Drawing for the job (mm, zero at the part's lowest x, y, z). A direction names the side the tool comes from. Round coordinates to 2 decimals unless told otherwise and drop trailing zeros. Write each loop counter-clockwise with the first axis right and the second up, starting at its lowest first coordinate (ties: lowest second). Pieces come first, ordered by that corner, then holes.
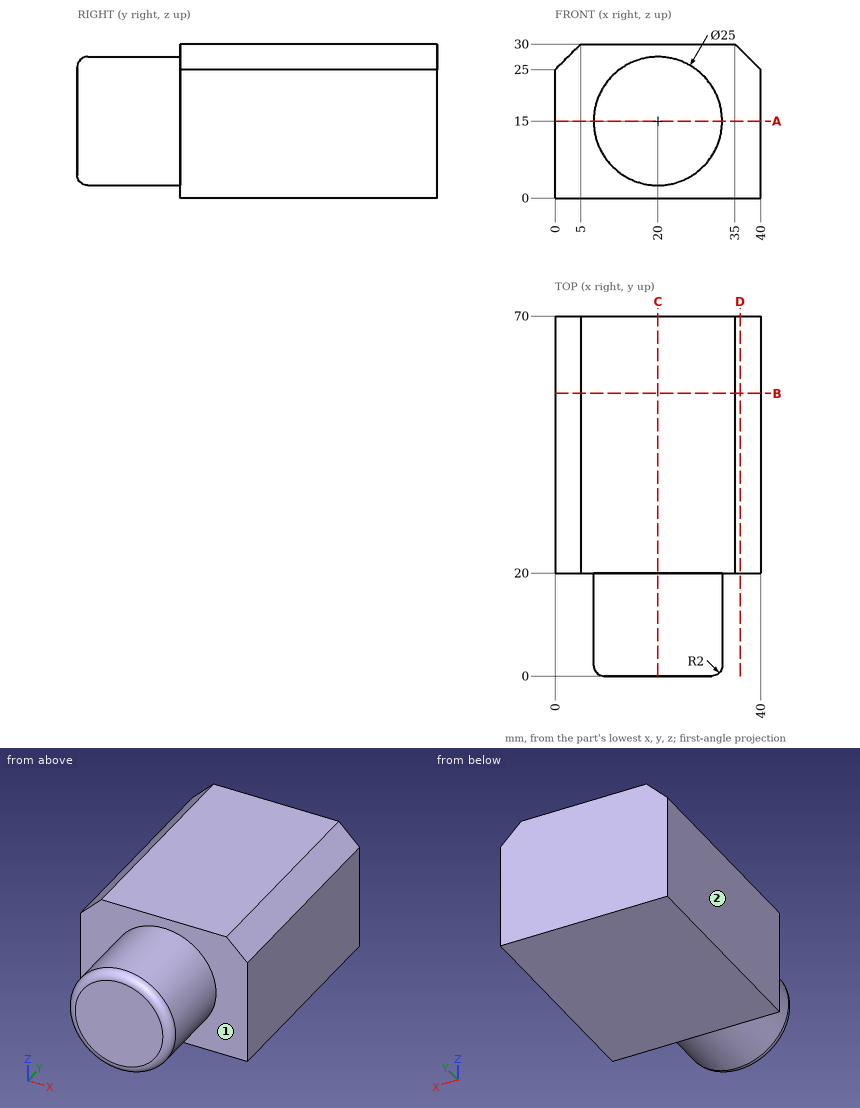
Q1. Tool access for the marked faces 1 and 2: list every direction of +Z, -Z, +X, -X, +Y, -Y with a clear straight run to the whole face (end or side of a thin tool).
Q2. Drop a flat-ended pin along its axis: P1, Ø1, axis at y = 7.5, z = 11.5, coming from the -X side. Give the stop position or say it passes through.
Q3. Saw through at D-D, the plane x = 36. Write the cut outline in (y, z), and give its area (3 significant figures).
Q4. Saw through at B-B, the plane y = 55. Write the cut outline in (x, z), and give its area (4 significant figures).
Q5. Saw through at A-A, the plane z = 15. Write the cut outline in (x, y), and give its area (3 significant figures).
Q6. Saw through at C-C, the plane x = 20. Write the cut outline in (y, z), and give its area (3 significant figures).
Q7. Wall check: line 1 (Y direction, x = 5, z = 7.75); line 2 (Y direction, x = 20.5, z = 26.5); line 3 (Z direction, x = 11.5, y = 10). Give the ranges that are in metal, low to high.
Computed:
1. face 1: -Y
1. face 2: +Z, -Z, -X, +Y, -Y
2. P1: stops at x = 7.87
3. outline: (20, 0) - (70, 0) - (70, 29) - (20, 29) - close
3. area: 1,450 mm2
4. outline: (0, 0) - (40, 0) - (40, 25) - (35, 30) - (5, 30) - (0, 25) - close
4. area: 1,175 mm2
5. outline: (0, 20) - (7.5, 20) - (7.5, 2) arc R2 ccw to (9.5, 0) - (30.5, 0) arc R2 ccw to (32.5, 2) - (32.5, 20) - (40, 20) - (40, 70) - (0, 70) - close
5. area: 2,500 mm2
6. outline: (0, 4.5) arc R2 ccw to (2, 2.5) - (20, 2.5) - (20, 0) - (70, 0) - (70, 30) - (20, 30) - (20, 27.5) - (2, 27.5) arc R2 ccw to (0, 25.5) - close
6. area: 2,000 mm2
7. line 1: y = 20 to 70
7. line 2: y = 0.27 to 70
7. line 3: z = 5.83 to 24.17
